```python
from build123d import *

# Parameters (mm, degrees)
F0_W     = 7.112
F0_H     = 7.366
F0_W_2   = 8.636
F0_H_2   = 9.652
F4_R     = 10.92
F5_DEPTH = 25.4
F6_R     = 8.128
F7_DEPTH = 16.51


with BuildPart() as f1:
    # F0 (on Front) → F1 (revolve)
    with BuildSketch(Plane.XZ):
        Polygon((-38.397264, 16), (-38.397264, 0), (-11.219264, 0), (-11.219264, 10.414), (-11.219264, 16), align=None)
    revolve(axis=Axis((-8.996764, 0, 0), (1, 0, 0)))

    # F0 (on Front) → F2 (revolve)
    with BuildSketch(Plane.XZ):
        Polygon((-11.219264, 10.414), (-11.219264, 0), (-6.139264, 0), (-6.139264, 7.366), (-6.139264, 10.414), align=None)
    revolve(axis=Axis((-8.996764, 0, 0), (1, 0, 0)))

    # F0 (on Front) → F3 (revolve)
    with BuildSketch(Plane.XZ):
        Polygon((0.972736, 7.366), (0.972736, 0), (18.752736, 0), (18.752736, 17.907), (0.972736, 17.907), align=None)
        Polygon((18.752736, 17.907), (18.752736, 0), (20.403736, 0), (22.054736, 0), (22.054736, 7.62), (22.054736, 19.558), (18.752736, 19.558), align=None)
        with Locations((-2.583264, 3.683)):
            Rectangle(F0_W, F0_H)
        Polygon((22.054736, 7.62), (22.054736, 0), (22.72404, 0), (41.33619, 0), (41.33619, 7.62), align=None)
        Polygon((41.33619, 7.62), (41.33619, 0), (44.660736, 0), (44.660736, 10.16), (41.358736, 7.62), align=None)
        Polygon((44.660736, 10.16), (44.660736, 0), (56.852736, 0), (56.852736, 9.652), (56.852736, 10.16), align=None)
        with Locations((61.170736, 4.826)):
            Rectangle(F0_W_2, F0_H_2)
    revolve(axis=Axis((-8.996764, 0, 0), (1, 0, 0)))

    # F4 (on face) → F5 (cut)
    with BuildSketch(Plane(origin=(-38.397264, 0, 0), x_dir=(0, -1, 0), z_dir=(-1, 0, 0))):
        Circle(F4_R)
    extrude(amount=-F5_DEPTH, mode=Mode.SUBTRACT)

    # F6 (on face) → F7 (cut)
    with BuildSketch(Plane.YZ.offset(65.488736)):
        Circle(F6_R)
    extrude(amount=-F7_DEPTH, mode=Mode.SUBTRACT)


solid = f1.part
```
Can you work these out from the model? Positions are in its coordinate system, mm. A direction names the side the tool comes from. Give positions to 0.01 mm unless a question says otherwise; leave off trailing zeros. Order: outer loops, then holes, each group sorted by start corner. A loop starts at its lowest first (then second) coordinate and runs counter-clockwise, first axis right, second up. Notation, with made-up numbers: M 73.5,74 L 116.5,74 A21 ccw 116.5,111 Z; hole C -5,52 d5. An arc over 180 degrees is marked long. One line per item, written item: value.
1) We'd pull the mould along Z, two halves only. Please class faces 1 (the face through (41.519, 4.712, -6.145)), 2 (the face through (22.055, 0, -8)), 3 (the face through (57.349, -1.762, -7.935)): released by +Z, released by -Z, zero draft, split by the parting line, or undercut.
Answer sheet:
face 1: split by the parting line
face 2: zero draft
face 3: undercut
2) For P1, Ø13, axis at y = 0, z = 0, coming from the +X side; P2, Ø5, axis at x = -3.5, z = -8, coming from the -Y side; P3, Ø10, axis at x = 1.5, y = 13.5, coming from the +Z side, each with a flat end and sliding along its axis, tell me the tip position at first contact or that it passes through.
Answer sheet:
P1: stops at x = 48.98
P2: stops at y = -4.9
P3: stops at z = 15.76
3) On a 3-axis mill with a long thin cutter (end or side, diameter ignored), from which of +Z, -Z, +X, -X, +Y, -Y can I reach the whole of each face in a straight line? I mean faces 4 (the face through (-25.875, -10.416, 3.28)), 5 (the face through (-8.715, -3.128, 9.933)), 6 (the face through (61.23, 5.87, -7.66)). Say none if no direction works.
Answer sheet:
face 4: -X
face 5: none
face 6: +X
4) I want a section at B-B, the plane x = 25.5. List the corners of the cut face in (y, z) for me, plus the area to 3 significant figures.
Answer sheet:
outline: C 0,0 d15.24
area: 182 mm^2
5) I want a section at C-C, the plane x = 12.5. List the corners of the cut face in (y, z) for me, plus the area to 3 significant figures.
Answer sheet:
outline: C 0,0 d35.81
area: 1,010 mm^2
6) I want a section at A-A, the plane y = 12. List the corners of the cut face in (x, z) for me, plus the area to 3 significant figures.
Answer sheet:
outline: M -38.4,-10.58 L -11.22,-10.58 L -11.22,10.58 L -38.4,10.58 Z; M 0.97,-13.29 L 18.75,-13.29 L 18.75,-15.44 L 22.05,-15.44 L 22.05,15.44 L 18.75,15.44 L 18.75,13.29 L 0.97,13.29 Z
area: 1,150 mm^2
7) Please list where these lines run through material, in increasing order: line 1 along X through (y, z) = (8.5, -8); line 2 along X through (y, z) = (8.5, 2); line 3 along X through (y, z) = (5.5, -5.5).
Answer sheet:
line 1: x = -38.4 to -11.22, 0.97 to 22.05
line 2: x = -13 to -6.14, 0.97 to 22.05, 42.8 to 65.49
line 3: x = -13 to -6.14, 0.97 to 22.05, 41.56 to 48.98
